Could you check a few things on this model? Use its own coordinates, in mm. A direction names the side the tool comes from. Coordinates: 2 decimals unless noted, no trailing zeros. Order: outer loops, then holes, each group sorted by start corner. A loop starts at its lowest first (then second) coordinate and runs counter-clockwise, first axis right, second up. Notation, with made-up numbers: (76, -31) -> (80, -31) arc R29 ccw to (80, -9) -> close; hole circle Ø8 at (88, -25.5). An arc over 180 degrees is marked (long way). Use a Markdown table: item, result. Add a question column.
1) Which directions (+Z, -Z, +X, -X, +Y, -Y) give clear straight access to the entire face, cutting with the end or side of a thin tool? Please do faces 5 (the flat face through (4, 2, 0)), 6 (the flat face through (108, 2, -7)).
2) If we section it at B-B (y = 0.95): Write out the boundary of the cut face in (x, z), plus the area to 3 significant figures.
3) Thinking about a two-plate mould opening in X: for faces 1 (the flat face through (59, 2, -15)), 2 (the flat face through (0, 2, -11)), 3 (the flat face through (59, 0, -16)), 4 (the flat face through (8, 2, -8)), which applies, +X half, -X half, draft (parallel to the pull), parting line (faces both ways), or undercut?
4) If we section it at A-A (z = -14): Write out the boundary of the cut face in (x, y), plus the area to 3 significant figures.
5) Will this pin go through, and if not, where does the flat tip stop? pin 1 Ø2 at (x, y) = (58.5, 3) entering from +Z.
6) If we section it at C-C (x = 54.5): Write out the boundary of the cut face in (y, z), plus the area to 3 significant figures.
7) If I drill on L1, parallel to X at y = 1, z = -14.25; L2, parallel to Z at x = 61, y = 3.6, over which ranges is the centre line in solid material (lowest first)? Write a range as [from, to].
Autodesk Inventor part; units mm, degrees
ref_plane "YZ Plane" through (0, 0, 0) normal (1, 0, 0) x (0, 1, 0)
ref_plane "XZ Plane" through (0, 0, 0) normal (0, 1, 0) x (-1, 0, 0)
ref_plane "XY Plane" through (0, 0, 0) normal (0, 0, 1) x (1, 0, 0)
sketch "Sketch1" plane through (0, 0, 0) normal (0, 1, 0) x (-1, 0, 0)
  line L0 (0, 0) -> (0, -15)
  line L1 (0, -15) -> (0, -23)
  line L2 (0, -23) -> (-116, -23)
  line L3 (-116, -23) -> (-116, -15)
  line L4 (-116, -15) -> (-116, 0)
  line L5 (-116, 0) -> (-108, 0)
  line L6 (-108, 0) -> (-108, -15)
  line L7 (-108, -15) -> (-8, -15)
  line L8 (-8, -15) -> (-8, 0)
  line L9 (-8, 0) -> (0, 0)
  dimension "d243" = 8
  dimension "d245" = 100
  dimension "d246" = 15
extrude "Extrusion1" add sketch "Sketch1" along normal blind 4
properties part number "Langbektang houder"
Answer sheet:
| question | item | result |
|---|---|---|
| 1 | face 5 | +Z, +X, -X, +Y, -Y |
| 1 | face 6 | +Z, +Y, -Y |
| 2 | outline | (0, -23) -> (116, -23) -> (116, 0) -> (108, 0) -> (108, -15) -> (8, -15) -> (8, 0) -> (0, 0) -> close |
| 2 | area | 1,170 mm2 |
| 3 | face 1 | undercut |
| 3 | face 2 | -X half |
| 3 | face 3 | draft |
| 3 | face 4 | undercut |
| 4 | outline | (0, 0) -> (8, 0) -> (8, 4) -> (0, 4) -> close; (108, 0) -> (116, 0) -> (116, 4) -> (108, 4) -> close |
| 4 | area | 64.0 mm2 |
| 5 | pin 1 | z = -15 |
| 6 | outline | (0, -23) -> (4, -23) -> (4, -15) -> (0, -15) -> close |
| 6 | area | 32.0 mm2 |
| 7 | L1 | [0, 8], [108, 116] |
| 7 | L2 | [-23, -15] |
